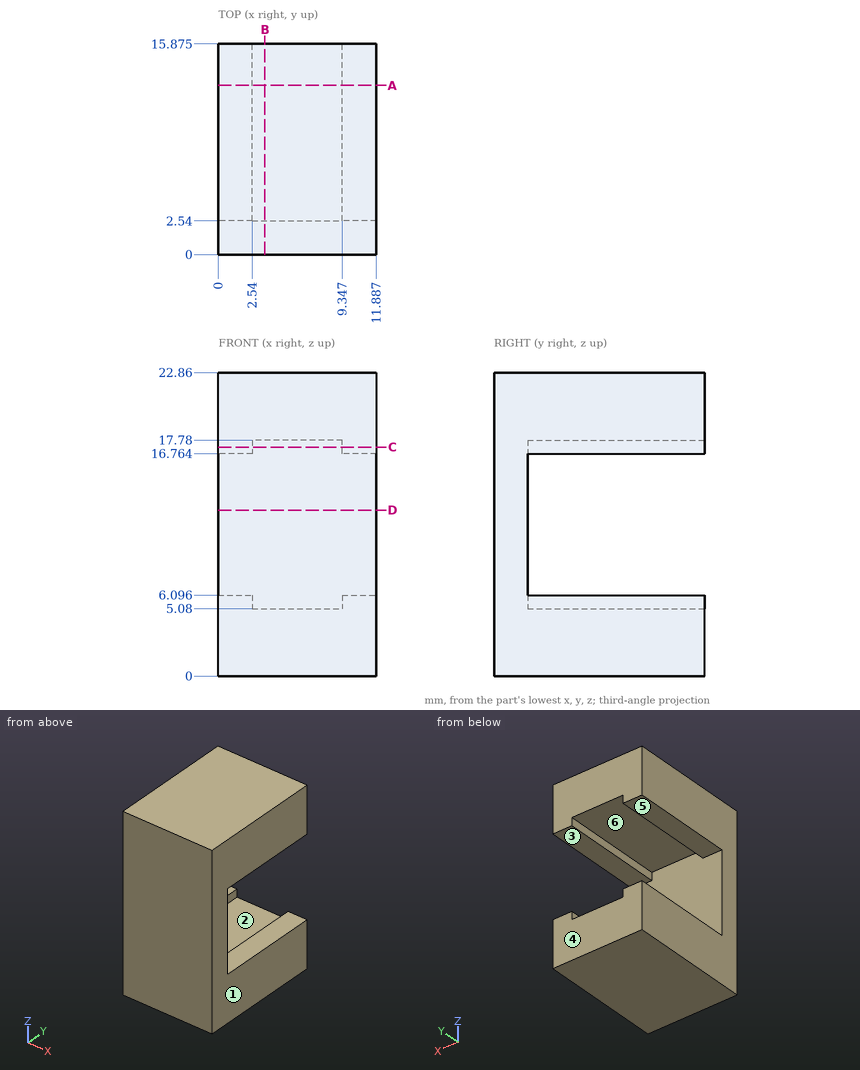
Check sheet for the drawn part. Datum: minimum x, y, z corner. Units: mm. A direction names the side the tool comes from. Give positions to 0.01 mm unless a question says otherwise; leave off trailing zeros. Loops run counter-clockwise (first coordinate to the right, second up) from the corner with the lowest first, then second, coordinate; pieces in that order, holes last.
1) Draft check along X on the marked faces 1, 2 and 3. Enter one of: pulls with the +X half, pulls with the -X half, needs draft (parallel to the pull), parting line crosses it, or undercut.
2) Sectioned sample at C-C, the plane z = 17.25. Enter the section's corners in (x, y) (1 decimal).
3) Sectioned sample at B-B, the plane x = 3.5. Enter the section's corners in (y, z) (3 decimals), then the cut area to 3 significant figures.
4) Thickness scan on line 1 along Z through (x, y) = (3.5, 3.75); line 2 along Z through (x, y) = (10.25, 13); line 3 along Y through (x, z) = (1.75, 15.25). Record the ranges inside material, lowest first.
5) Set-up check for the marked faces 4, 5 and 6: record each of +Z, -Z, +X, -X, +Y, -Y from which the full face is reachable in a straight line by a thin tool's end or side.
6) Sectioned sample at D-D, the plane z = 12.5. Enter the section's corners in (x, y).
7) Sectioned sample at A-A, the plane y = 12.75. Enter the section's corners in (x, z), then the cut area to 3 significant figures.
8) Depth check by flat-ended pin: pin 1 Ø1 at (x, z) = (8.5, 11) entering from +Y. Enter the tip coordinate at first touch or a pass-through.
Answers:
1. face 1: pulls with the +X half
1. face 2: undercut
1. face 3: needs draft
2. outline: (0, 0) - (11.9, 0) - (11.9, 15.9) - (9.3, 15.9) - (9.3, 2.5) - (2.5, 2.5) - (2.5, 15.9) - (0, 15.9) - close
3. outline: (0, 0) - (15.875, 0) - (15.875, 5.08) - (2.54, 5.08) - (2.54, 17.78) - (15.875, 17.78) - (15.875, 22.86) - (0, 22.86) - close
3. area: 194 mm2
4. line 1: z = 0 to 5.08, 17.78 to 22.86
4. line 2: z = 0 to 6.1, 16.76 to 22.86
4. line 3: y = 0 to 2.54
5. face 4: +Z, -Z, +X, -X, +Y
5. face 5: +X, -X, +Y
5. face 6: +Y
6. outline: (0, 0) - (11.89, 0) - (11.89, 2.54) - (0, 2.54) - close
7. outline: (0, 0) - (11.89, 0) - (11.89, 6.1) - (9.35, 6.1) - (9.35, 5.08) - (2.54, 5.08) - (2.54, 6.1) - (0, 6.1) - close; (0, 16.76) - (2.54, 16.76) - (2.54, 17.78) - (9.35, 17.78) - (9.35, 16.76) - (11.89, 16.76) - (11.89, 22.86) - (0, 22.86) - close
7. area: 131 mm2
8. pin 1: stops at y = 2.54
